Work out the finished part from the listing and answer in its coordinate system (mm). Face numbers are marked on the shaded views. A direction names the side the tool comes from. Round coordinates to 2 decimals unless told otherwise and drop trailing zeros. Order: outer loops, then holes, each group sorted by start corner. A loop starts at its lowest first (then second) coordinate and runs counter-clockwise, first axis right, second up. Notation, with made-up numbers: (37.5, 89.25) - (85.5, 89.25) arc R24 ccw to (85.5, 113.25) - close; hole circle Ø6 at (46, -19.75). An arc over 180 degrees is marked (long way). Answer in a Markdown table with one row per item.
from build123d import *
from build123d.topology import SkipClean

# Parameters (mm, degrees)
SKETCH1_W                = 25.809397514
SKETCH1_H                = 25.809397514
BOSS_EXTRUDE1_DEPTH      = 28.6
BOSS_EXTRUDE3_DEPTH      = 28.6
CUT_EXTRUDE4_DEPTH       = 42.564184101
CUT_EXTRUDE4_DEPTH_BACK  = 42.564184101
SKETCH4_R                = 14.25
SKETCH5_R                = 14.25
SKETCH5_R_2              = 14
BOSS_EXTRUDE4_DEPTH      = 20
SKETCH6_R                = 7.705
BOSS_EXTRUDE5_DEPTH      = 2.27
SKETCH7_R                = 5
CUT_EXTRUDE5_DEPTH       = 5
BOSS_EXTRUDE7_REACH      = 66.131
BOSS_EXTRUDE7_END_RADIUS = 18.25
BOSS_EXTRUDE7_START      = 20
SKETCH8_R                = 7.705
CUT_EXTRUDE8_DEPTH       = 57.696759272
CUT_EXTRUDE8_DEPTH_BACK  = 57.696759272
SKETCH12_R               = 5


with BuildPart() as part:
    # Sketch1 → Boss-Extrude1 (new body)
    with BuildSketch(Plane(origin=(0, 0, 0), x_dir=(1, 0, 0), z_dir=(0, 1, 0))):
        Rectangle(SKETCH1_W, SKETCH1_H)
    extrude(amount=BOSS_EXTRUDE1_DEPTH)

    # Sketch2 → Revolve1 (revolve)
    with BuildSketch(Plane.ZY):
        Polygon((0, 0), (0, -3.98), (11, -3.98), (18.25, 0), align=None)
    revolve1 = revolve(axis=Axis((0, 0, 0), (0, -1, 0)))

    # Mirror2: Revolve1 across plane
    add(revolve1.mirror(Plane(origin=(0, 14.3, 0), x_dir=(0, 0, 1), z_dir=(0, -1, 0))))

    # Sketch1_4 → Boss-Extrude3 (add)
    with BuildSketch(Plane(origin=(0, 0, 0), x_dir=(1, 0, 0), z_dir=(0, 1, 0))):
        with BuildLine():
            Line((-12.904698757, -12.904698757), (-12.904698757, 12.904698757))
            ThreePointArc((-12.904698757, 12.904698757), (-18.25, 0), (-12.904698757, -12.904698757))
        make_face()
        with BuildLine():
            ThreePointArc((12.904698757, 12.904698757), (0, 18.25), (-12.904698757, 12.904698757))
            Line((-12.904698757, 12.904698757), (12.904698757, 12.904698757))
        make_face()
        with BuildLine():
            ThreePointArc((18.25, 0), (16.860801468, 6.983972641), (12.904698757, 12.904698757))
            Line((12.904698757, 12.904698757), (12.904698757, -12.904698757))
            ThreePointArc((12.904698757, -12.904698757), (16.860801468, -6.983972641), (18.25, 0))
        make_face()
        with BuildLine():
            Line((12.904698757, -12.904698757), (-12.904698757, -12.904698757))
            ThreePointArc((-12.904698757, -12.904698757), (0, -18.25), (12.904698757, -12.904698757))
        make_face()
    extrude(amount=BOSS_EXTRUDE3_DEPTH)

    # Sketch4 → Cut-Extrude4 (cut, two sides: drawn at the far end of the back side and taken through both)
    with SkipClean():  # the faces are left unmerged after this step: merging them gives an invalid solid
        with BuildSketch(Plane.ZY.offset(-CUT_EXTRUDE4_DEPTH_BACK)):
            with Locations((0, 14.3)):
                Circle(SKETCH4_R)
        extrude(amount=CUT_EXTRUDE4_DEPTH + CUT_EXTRUDE4_DEPTH_BACK, mode=Mode.SUBTRACT)

    # Sketch5 → Boss-Extrude4 (add, symmetric)
    with SkipClean():  # the faces are left unmerged after this step: merging them gives an invalid solid
        with BuildSketch(Plane.ZY):
            with Locations(Location((0, 14.3, 0), (0, 0, 180))):
                Circle(SKETCH5_R)
            with Locations((0, 14.3)):
                Circle(SKETCH5_R_2, mode=Mode.SUBTRACT)
        extrude(amount=BOSS_EXTRUDE4_DEPTH, both=True)

    # Sketch6 → Boss-Extrude5 (add)
    with SkipClean():  # the faces are left unmerged after this step: merging them gives an invalid solid
        with BuildSketch(Plane(origin=(0, 32.58, 0), x_dir=(1, 0, 0), z_dir=(0, 1, 0))):
            with Locations(Location((0, 0, 0), (0, 0, 270))):
                Circle(SKETCH6_R)
        extrude(amount=BOSS_EXTRUDE5_DEPTH)

    # Sketch7 → Cut-Extrude5 (cut)
    with SkipClean():  # the faces are left unmerged after this step: merging them gives an invalid solid
        with BuildSketch(Plane(origin=(0, 34.85, 0), x_dir=(1, 0, 0), z_dir=(0, 1, 0))):
            with Locations(Location((0, 0, 0), (0, 0, 270))):
                Circle(SKETCH7_R)
        extrude(amount=-CUT_EXTRUDE5_DEPTH, mode=Mode.SUBTRACT)

    # Boss-Extrude7: up to this cylinder (the profile starts outside it)
    with SkipClean():  # the faces are left unmerged after this step: merging them gives an invalid solid
        boss_extrude7_end = Plane(origin=(0, 14.3, 0), z_dir=(0, -1, 0)) * Cylinder(BOSS_EXTRUDE7_END_RADIUS, 169.762, mode=Mode.PRIVATE)
        # Sketch8 → Boss-Extrude7 (add, up to the surface)
        with BuildSketch(Plane.XY.offset(BOSS_EXTRUDE7_START), mode=Mode.PRIVATE) as boss_extrude7_sk1:
            with Locations((0, 14.3)):
                Circle(SKETCH8_R)
        boss_extrude7_tool1 = extrude(boss_extrude7_sk1.sketch, amount=-BOSS_EXTRUDE7_REACH, mode=Mode.PRIVATE) - boss_extrude7_end
        boss_extrude7 = boss_extrude7_tool1.solids().sort_by_distance((0, 14.3, 20))[0]
        add(boss_extrude7)

    # Mirror5: Boss-Extrude7 across plane
    with SkipClean():  # the faces are left unmerged after this step: merging them gives an invalid solid
        add(boss_extrude7.mirror(Plane.XY))

    # Sketch12 → Cut-Extrude8 (cut, two sides: drawn at the far end of the back side and taken through both)
    with SkipClean():  # the faces are left unmerged after this step: merging them gives an invalid solid
        with BuildSketch(Plane.XY.offset(20).offset(-CUT_EXTRUDE8_DEPTH_BACK)):
            with Locations((0, 14.3)):
                Circle(SKETCH12_R)
        extrude(amount=CUT_EXTRUDE8_DEPTH + CUT_EXTRUDE8_DEPTH_BACK, mode=Mode.SUBTRACT)


solid = part.part
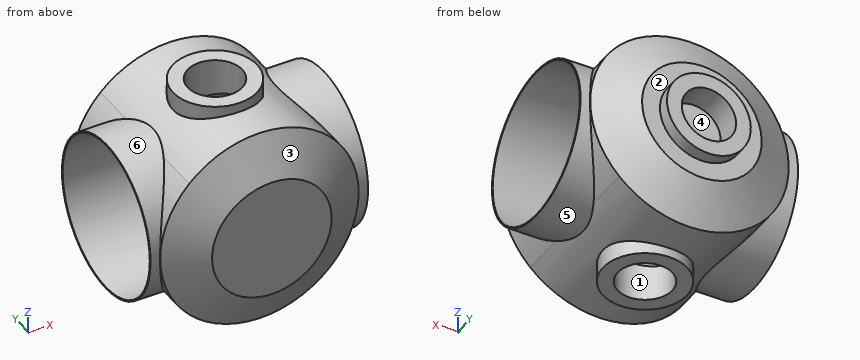
1) The mould has two halves that part along X. Classify the marked faces 1, 2 and 3: released by +X, released by -X, zero draft, split by the parting line, or undercut.
Filled in:
| item | result |
|---|---|
| face 1 | undercut |
| face 2 | zero draft |
| face 3 | split by the parting line |
2) Which of the six approach directions +Z, -Z, +X, -X, +Y, -Y give full straight-line access (tool end or side, diameter ignored) to the marked faces 4, 5 and 6?
Filled in:
| item | result |
|---|---|
| face 4 | +Y |
| face 5 | +X |
| face 6 | -X |
3) Find section C-C, the plane y = 24.5. Give the vertices of the cut face in (x, z).
Filled in:
| item | result |
|---|---|
| outline | (-20, -9.95) - (-15.3, -9.95) arc R18.25 ccw to (15.3, -9.95) - (20, -9.95) - (20, -9.59) - (-20, -9.59) - close; (-20, 9.59) - (20, 9.59) - (20, 9.95) - (15.3, 9.95) arc R18.25 ccw to (-15.3, 9.95) - (-20, 9.95) - close |
4) Find the intervals of material crossed by probe 1 along X at (y, z) = (14.3, 17) (3 decimals); probe 2 along Z at (x, y) = (-13.5, 14.5); probe 3 along Y at (x, z) = (-2.5, 0), in increasing order. Write a range as from..to.
Filled in:
| item | result |
|---|---|
| probe 1 | x = -7.705..-5, 5..7.705 |
| probe 2 | z = -14.25..-14, 14..14.25 |
| probe 3 | y = -3.98..0.3, 28.3..29.85 |
5) Each of these flat-tipped pins is pushed along its axis until it touches: pin 1 (12 mm diameter, centred on y = 6, z = -14, fed in from -X); pin 2 (22.5 mm diameter, centred on y = 14.3, z = 0, fed in from +X); pin 3 (1.5 mm diameter, centred on x = -6.5, z = -13.5, fed in from +Y) (3 decimals); pin 4 (8 mm diameter, centred on x = -8.5, y = 23.5, fed in from +Z). Where does it stop, or does it pass through?
Filled in:
| item | result |
|---|---|
| pin 1 | stops at x = -20 |
| pin 2 | passes through |
| pin 3 | stops at y = 30.805 |
| pin 4 | stops at z = 17.69 |
6) Find section A-A, the plane y = 14.3. Give the vertices of the cut face in (x, z) (3 decimals).
Filled in:
| item | result |
|---|---|
| outline | (-20, -14.25) - (-11.402, -14.25) arc R18.25 ccw to (-7.705, -16.544) - (-7.705, -20) - (-5, -20) - (-5, -14) - (-20, -14) - close; (-20, 14) - (-5, 14) - (-5, 20) - (-7.705, 20) - (-7.705, 16.544) arc R18.25 ccw to (-11.402, 14.25) - (-20, 14.25) - close; (5, -20) - (7.705, -20) - (7.705, -16.544) arc R18.25 ccw to (11.402, -14.25) - (20, -14.25) - (20, -14) - (5, -14) - close; (5, 14) - (20, 14) - (20, 14.25) - (11.402, 14.25) arc R18.25 ccw to (7.705, 16.544) - (7.705, 20) - (5, 20) - close |
